Here's how the part is built. I have some questions about the finished solid (model axes, mm). A direction names the side the tool comes from. Round coordinates to 2 decimals unless told otherwise and drop trailing zeros. Loops run counter-clockwise (first coordinate to the right, second up) from the corner with the lowest first, then second, coordinate; pieces in that order, holes last. Notation, with made-up numbers: M 35.25,66.25 L 59.25,66.25 A30 ccw 59.25,96.25 Z; hole C 15.5,53.5 d9. An arc over 180 degrees is marked long. Answer as a JSON object with one key per item and string values.
from build123d import *
from OCP.BRepFilletAPI import BRepFilletAPI_MakeChamfer

# Parameters (mm, degrees)
EXTRUDE_1_DEPTH     = 10
EXTRUDE_1_2_DEPTH   = 10
EXTRUDE_1_3_DEPTH   = 10
EXTRUDE_1_4_DEPTH   = 10
EXTRUDE_2_DEPTH     = 2.5
EXTRUDE_3_DEPTH     = 10
CUT_EXTRUDE_1_DEPTH = 6
FILLET_4_R          = 1
FILLET_5_R          = 0.5
CUT_EXTRUDE_2_DEPTH = 50.301485276
CHAMFER_1_SIZE      = 1.5
CHAMFER_1_SIZE2     = 1.532867746
CHAMFER_1_SIZE2_2   = 1.505273584
CHAMFER_2_SIZE      = 1.5
CHAMFER_2_SIZE2     = 4.152297663


with BuildPart() as part:
    # Sketch 1 → Extrude 1 (new body)
    with BuildSketch(Plane(origin=(0, 0, 0), x_dir=(1, 0, 0), z_dir=(0, 1, 0))):
        Polygon((-7.6, 13.163586138), (-7.6, 28.261662349), (-10.6, 28.261662349), (-10.6, 18.35973856), (-27.750635095, 28.261662349), (-29.250635095, 25.663586138), align=None)
    extrude(amount=EXTRUDE_1_DEPTH)



with BuildPart() as body_2:
    # Sketch 1 → Extrude 1 2 (new body)
    with BuildSketch(Plane(origin=(0, 0, 0), x_dir=(1, 0, 0), z_dir=(0, 1, 0))):
        Polygon((-36.850635095, 12.5), (-7.6, -4.387862046), (-7.6, -24.387862046), (-10.6, -24.387862046), (-10.6, -7.048921698), (-38.414383917, 9.939787192), align=None)
    extrude(amount=EXTRUDE_1_2_DEPTH)


with BuildPart() as body_3:
    # Sketch 1 → Extrude 1 3 (new body)
    with BuildSketch(Plane(origin=(0, 0, 0), x_dir=(1, 0, 0), z_dir=(0, 1, 0))):
        Polygon((7.6, -24.387862046), (7.6, -4.387862046), (36.850635095, 12.5), (38.414383917, 9.939787192), (10.6, -7.048921698), (10.6, -24.387862046), align=None)
    extrude(amount=EXTRUDE_1_3_DEPTH)


with BuildPart() as body_4:
    # Sketch 1 → Extrude 1 4 (new body)
    with BuildSketch(Plane(origin=(0, 0, 0), x_dir=(1, 0, 0), z_dir=(0, 1, 0))):
        Polygon((29.250635095, 25.663586138), (7.6, 13.163586138), (7.6, 28.261662349), (10.6, 28.261662349), (10.6, 18.35973856), (27.750635095, 28.261662349), align=None)
    extrude(amount=EXTRUDE_1_4_DEPTH)


with BuildPart() as part_1:
    add(part.part)

    add(body_2.part)  # Extrude 2 merges body 2

    add(body_3.part)  # Extrude 2 merges body 3

    add(body_4.part)  # Extrude 2 merges body 4
    # Sketch 2 → Extrude 2 (add)
    with BuildSketch(Plane.XZ):
        Polygon((-10.6, 24.387862046), (10.6, 24.387862046), (10.6, 7.048921698), (38.414383917, -9.939787192), (27.750635095, -28.261662349), (-27.750635095, -28.261662349), (-38.414383917, -9.939787192), (-10.6, 7.048921698), align=None)
    extrude(amount=EXTRUDE_2_DEPTH)

    # Sketch 3 → Extrude 3 (add)
    with BuildSketch(Plane(origin=(0, 0, 0), x_dir=(1, 0, 0), z_dir=(0, 1, 0))):
        Polygon((9.158845727, 14.063586138), (16.758845727, 0.9), (7.6, -4.387862046), (7.6, 13.163586138), align=None)
        Polygon((-7.6, -4.387862046), (-7.6, 13.163586138), (-9.158845727, 14.063586138), (-16.758845727, 0.9), align=None)
    extrude(amount=EXTRUDE_3_DEPTH)

    # Sketch 4 → Cut-Extrude 1 (cut)
    with BuildSketch(Plane(origin=(0, 10, 0), x_dir=(1, 0, 0), z_dir=(0, 1, 0))):
        Polygon((-15.887237696, 6.285749615), (-6.628889419, 0.940439745), (-4.128889419, 5.270566763), (-13.387237696, 10.615876634), align=None)
        Polygon((14.008406819, 10.974508794), (3.507720297, 4.911934604), (6.007720297, 0.581807585), (16.508406819, 6.644381775), align=None)
    extrude(amount=-CUT_EXTRUDE_1_DEPTH, mode=Mode.SUBTRACT)

    # Fillet 4
    fillet_4_edges = [part_1.edges().sort_by_distance(p)[0] for p in [
        (-14.208845727, 7, -5.316729559),
        (14.208845727, 7, -5.316729559),
        (-7.6, 7, -1.5011107),
        (7.6, 7, -1.5011107),
    ]]
    fillet(fillet_4_edges, radius=FILLET_4_R)

    # Fillet 5
    fillet_5_edges = [part_1.edges().sort_by_distance(p)[0] for p in [
        (-11.708845727, 7, -9.646856578),
        (11.708845727, 7, -9.646856578),
        (-7.6, 7, -7.274613392),
        (7.6, 7, -7.274613392),
    ]]
    fillet(fillet_5_edges, radius=FILLET_5_R)

    # Sketch 5 → Cut-Extrude 2 (cut, through all)
    with BuildSketch(Plane(origin=(0, 10, 0), x_dir=(1, 0, 0), z_dir=(0, 1, 0))):
        Polygon((-24.047037107, 33.630998613), (-39.832865352, 6.508644255), (-44.756690746, 10.727475508), (-28.61540602, 34.978771584), align=None)
        Polygon((24.284000657, 33.223860688), (39.70321054, 6.731410124), (44.299549415, 9.406584081), (29.808170892, 34.304885099), align=None)
    extrude(amount=-CUT_EXTRUDE_2_DEPTH, mode=Mode.SUBTRACT)

    # Chamfer 1: one chamfer whose edges measure the first distance from different faces: ONE call of the kernel's chamfer builder (chamfer() names one face for all edges)
    chamfer_1_edges_1 = [part_1.edges().sort_by_distance(p)[0] for p in [
        (10.6, 5, -28.261662349),
        (-10.6, 3.75, 24.387862046),
        (10.6, 3.75, 24.387862046),
        (-10.6, 5, -28.261662349),
    ]]
    chamfer_1_edges_2 = [part_1.edges().sort_by_distance(p)[0] for p in [
        (-37.987585708, 3.75, -9.679103708),
    ]]
    chamfer_1_side_2 = [part_1.faces().sort_by_distance(p)[0] for p in [
        (-28.072162886, 9.751296174, -26.715245698),
    ]]
    chamfer_1_edges_3 = [part_1.edges().sort_by_distance(p)[0] for p in [
        (-27.317619745, 5, -28.01166082),
    ]]
    chamfer_1_side_3 = [part_1.faces().sort_by_distance(p)[0] for p in [
        (-28.072162886, 9.751296174, -26.715245698),
    ]]
    chamfer_1_edges_4 = [part_1.edges().sort_by_distance(p)[0] for p in [
        (27.317619745, 5, -28.01166082),
    ]]
    chamfer_1_side_4 = [part_1.faces().sort_by_distance(p)[0] for p in [
        (28.072162886, 9.751296174, -26.715245698),
    ]]
    chamfer_1_edges_5 = [part_1.edges().sort_by_distance(p)[0] for p in [
        (37.987585708, 3.75, -9.679103708),
    ]]
    chamfer_1_side_5 = [part_1.faces().sort_by_distance(p)[0] for p in [
        (28.072162886, 9.751296174, -26.715245698),
    ]]
    chamfer_1 = BRepFilletAPI_MakeChamfer(part_1.part.solid().wrapped)
    for e in chamfer_1_edges_1:
        chamfer_1.Add(CHAMFER_1_SIZE, e.wrapped)
    for e in chamfer_1_edges_2:
        chamfer_1.Add(CHAMFER_1_SIZE, CHAMFER_1_SIZE2, e.wrapped, chamfer_1_side_2[0].wrapped)  # the first distance lies on this face
    for e in chamfer_1_edges_3:
        chamfer_1.Add(CHAMFER_1_SIZE, CHAMFER_1_SIZE2_2, e.wrapped, chamfer_1_side_3[0].wrapped)  # the first distance lies on this face
    for e in chamfer_1_edges_4:
        chamfer_1.Add(CHAMFER_1_SIZE, CHAMFER_1_SIZE2_2, e.wrapped, chamfer_1_side_4[0].wrapped)  # the first distance lies on this face
    for e in chamfer_1_edges_5:
        chamfer_1.Add(CHAMFER_1_SIZE, CHAMFER_1_SIZE2, e.wrapped, chamfer_1_side_5[0].wrapped)  # the first distance lies on this face
    add(Compound.cast(chamfer_1.Shape()), mode=Mode.REPLACE)

    # Chamfer 2: one chamfer whose edges measure the first distance from different faces: ONE call of the kernel's chamfer builder (chamfer() names one face for all edges)
    chamfer_2_edges_1 = [part_1.edges().sort_by_distance(p)[0] for p in [
        (-27.172113158, -1.25, -28.261662349),
    ]]
    chamfer_2_side_1 = [part_1.faces().sort_by_distance(p)[0] for p in [
        (-28.449432149, 9.764143386, -26.067042101),
    ]]
    chamfer_2_edges_2 = [part_1.edges().sort_by_distance(p)[0] for p in [
        (27.172113158, -1.25, -28.261662349),
    ]]
    chamfer_2_side_2 = [part_1.faces().sort_by_distance(p)[0] for p in [
        (28.449432149, 9.764143386, -26.067042101),
    ]]
    chamfer_2 = BRepFilletAPI_MakeChamfer(part_1.part.solid().wrapped)
    for e in chamfer_2_edges_1:
        chamfer_2.Add(CHAMFER_2_SIZE, CHAMFER_2_SIZE2, e.wrapped, chamfer_2_side_1[0].wrapped)  # the first distance lies on this face
    for e in chamfer_2_edges_2:
        chamfer_2.Add(CHAMFER_2_SIZE, CHAMFER_2_SIZE2, e.wrapped, chamfer_2_side_2[0].wrapped)  # the first distance lies on this face
    add(Compound.cast(chamfer_2.Shape()), mode=Mode.REPLACE)


solid = part_1.part
Item 1: I'm going to push flat-ended pins straight in: pin 1 Ø2.5 at (y, z) = (5, -21) entering from +X; pin 2 Ø3.5 at (x, z) = (11.5, -5) entering from +Y; pin 3 Ø3 at (y, z) = (7, 0) entering from +X; pin 4 Ø6 at (x, y) = (-4, 4.5) entering from +Z. Where does each tip first touch, or does it pass through?
Resolved:
{"pin 1": "x = 23.34", "pin 2": "y = 10", "pin 3": "x = 24.6", "pin 4": "through"}
Item 2: On a 3-axis mill with a long thin cutter (end or side, diameter ignored), from which of +Z, -Z, +X, -X, +Y, -Y can I reach the whole of each face in a straight line? I mean faces 1 (the face through (9.84, 4.93, -27.52)), 2 (the face through (-10, 4, -6)), 3 (the face through (-27, 5, -27)), 4 (the face through (25.439, -1.267, -27.623)), 5 (the face through (-7.6, 3.8, -1.6)). Say none if no direction works.
Resolved:
{"face 1": "-Z, +Y", "face 2": "+Y", "face 3": "-Z, -X, +Y", "face 4": "-Z, +X, +Y, -Y", "face 5": "+Z, -Z, +Y"}
Item 3: I want a section at C-C, the plane x = -2. Please give me the cut outline in (y, z), then the cut area to 3 significant figures.
Resolved:
{"outline": "M -2.5,-28.26 L 0,-28.26 L 0,24.39 L -2.5,24.39 Z", "area": "132 mm²"}
Item 4: I want a section at D-D, the plane z = -24. Please give me the cut outline in (x, y), then the cut area to 3 significant figures.
Resolved:
{"outline": "M -29.65,-2.5 L 29.65,-2.5 L 29.65,0 L 26.37,0 L 26.37,10 L 20.37,10 L 20.37,0 L 10.6,0 L 10.6,10 L 7.6,10 L 7.6,0 L -7.6,0 L -7.6,10 L -10.6,10 L -10.6,0 L -20.37,0 L -20.37,10 L -26.37,10 L -26.37,0 L -29.65,0 Z", "area": "328 mm²"}
Item 5: Please list where these lines run through material, in increasing order: probe 1 along X at (y, z) = (7.5, 12); probe 2 along X at (y, z) = (3.5, -7); probe 3 along X at (y, z) = (8.25, -21.5). Write a range as from..to.
Resolved:
{"probe 1": "-10.6..-7.6, 7.6..10.6", "probe 2": "-33.6..-27.32, -13.24..-7.6, 7.6..13.24, 27.32..33.6", "probe 3": "-22.04..-16.04, -10.6..-7.6, 7.6..10.6, 16.04..22.04"}
Item 6: I want a section at B-B, the plane z = 8. Please give me the cut outline in (x, y).
Resolved:
{"outline": "M -10.6,-2.5 L 10.6,-2.5 L 10.6,10 L 7.6,10 L 7.6,0 L -7.6,0 L -7.6,10 L -10.6,10 Z"}
Item 7: If we mould it in two halves opening along X, with no side actions, what happens to faces 6 (the face through (14, 10, -20)), 7 (the face through (-18.199, 4.93, -22.747)), 8 (the face through (-9.86, 3.84, 23.63)), 9 (the face through (12.91, 3.82, -7.57))? For each: pulls with the +X half, pulls with the -X half, needs draft (parallel to the pull), parting line crosses it, or undercut.
Resolved:
{"face 6": "needs draft", "face 7": "undercut", "face 8": "pulls with the -X half", "face 9": "undercut"}
